```python
from build123d import *

# Parameters (mm, degrees)
SKETCH9_W           = 27.5
SKETCH9_H           = 28
BOSS_EXTRUDE2_DEPTH = 7.5
SKETCH10_W          = 23.5
SKETCH10_H          = 25.45
CUT_EXTRUDE1_DEPTH  = 6.1
SKETCH12_W          = 18.5
SKETCH12_H          = 12.3
CUT_EXTRUDE2_DEPTH  = 3
SKETCH11_W          = 9.585282086
SKETCH11_H          = 9.717675131
CUT_EXTRUDE3_DEPTH  = 5.05


with BuildPart() as part:
    # Sketch9 → Boss-Extrude2 (new, symmetric)
    with BuildSketch(Plane(origin=(0, 0, 0), x_dir=(1, 0, 0), z_dir=(0, 1, 0))):
        with Locations((0, 14)):
            Rectangle(SKETCH9_W, SKETCH9_H)
    extrude(amount=BOSS_EXTRUDE2_DEPTH, both=True)

    # Sketch10 → Cut-Extrude1 (cut, symmetric)
    with BuildSketch(Plane(origin=(0, 0, 0), x_dir=(1, 0, 0), z_dir=(0, 1, 0))):
        with Locations((0, 12.775)):
            Rectangle(SKETCH10_W, SKETCH10_H)
    extrude(amount=CUT_EXTRUDE1_DEPTH, both=True, mode=Mode.SUBTRACT)

    # Sketch12 → Cut-Extrude2 (cut)
    with BuildSketch(Plane.XY.offset(-28)):
        Rectangle(SKETCH12_W, SKETCH12_H)
    extrude(amount=CUT_EXTRUDE2_DEPTH, mode=Mode.SUBTRACT)

    # Sketch11 → Cut-Extrude3 (cut)
    with BuildSketch(Plane.XY.offset(5)):
        with Locations((8.957358957, -0.433824782)):
            Rectangle(SKETCH11_W, SKETCH11_H)
    extrude(amount=-CUT_EXTRUDE3_DEPTH, mode=Mode.SUBTRACT)


with BuildPart() as body_2:
    # Split1: the piece on the far side of the plane
    add(part.part)
    split(bisect_by=Plane.ZX, keep=Keep.BOTTOM)


with BuildPart() as part_1:
    add(part.part)

    # Split1
    split(bisect_by=Plane.ZX, keep=Keep.TOP)


solid = part_1.part
```
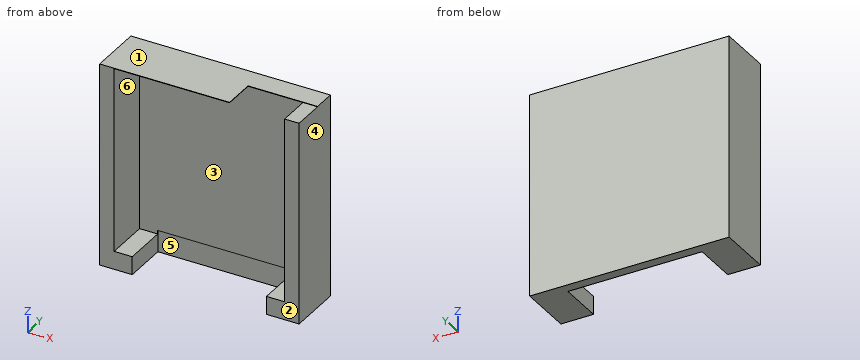
Check sheet for the modelled part. Datum: model origin and axes. Units: mm. Face numbers are marked on the shaded views. A direction names the side the tool comes from. Round coordinates to 2 decimals unless told otherwise and drop trailing zeros. Loops run counter-clockwise (first coordinate to the right, second up) from the corner with the lowest first, then second, coordinate; pieces in that order, holes last. Notation, with made-up numbers: (51, -29.75) -> (85, -29.75) arc R6 ccw to (85, -19.75) -> close; hole circle Ø6 at (1, -12). An arc over 180 degrees is marked (long way). Answer in a Markdown table with one row per item.
Q1. Release check for a two-part mould opening along Z. For the marked faces 1, 2 and 3 record: released by +Z, released by -Z, zero draft, split by the parting line, or undercut.
Data:
| item | result |
|---|---|
| face 1 | released by +Z |
| face 2 | zero draft |
| face 3 | undercut |
Q2. Thickness scan on L1, parallel to X at y = 4, z = -16.25; L2, parallel to Z at x = 10.75, y = 2; L3, parallel to Y at x = 1.75, z = -8.5. Record the ranges inside material, lowest first.
Data:
| item | result |
|---|---|
| L1 | x = -13.75 to -11.75, 11.75 to 13.75 |
| L2 | z = -28 to -25.5 |
| L3 | y = 6.1 to 7.5 |
Q3. Set-up check for the marked faces 4, 5 and 6: record each of +Z, -Z, +X, -X, +Y, -Y from which the full face is reachable in a straight line by a thin tool's end or side.
Data:
| item | result |
|---|---|
| face 4 | +Z, -Z, +X, +Y, -Y |
| face 5 | -Z, -Y |
| face 6 | -Y |
Q4. Sectioned sample at A-A on y = 4. Enter the section's corners in (x, z).
Data:
| item | result |
|---|---|
| outline | (-13.75, -28) -> (-9.25, -28) -> (-9.25, -25.5) -> (-11.75, -25.5) -> (-11.75, -0.05) -> (4.16, -0.05) -> (4.16, 0) -> (-13.75, 0) -> close; (9.25, -28) -> (13.75, -28) -> (13.75, -0.05) -> (11.75, -0.05) -> (11.75, -25.5) -> (9.25, -25.5) -> close |
Q5. Sectioned sample at C-C on z = -18.5. Enter the section's corners in (x, y).
Data:
| item | result |
|---|---|
| outline | (-13.75, 0) -> (-11.75, 0) -> (-11.75, 6.1) -> (11.75, 6.1) -> (11.75, 0) -> (13.75, 0) -> (13.75, 7.5) -> (-13.75, 7.5) -> close |
Q6. Go/stop test with flat-tipped pins: P1, Ø1.5, axis at x = 10.5, y = 2.5, coming from the +Z side; P2, Ø2, axis at x = -11, y = 3, coming from the +Z side; P3, Ø1.6, axis at x = 12.5, y = 1.5, coming from the +Z side; P4, Ø2, axis at x = 7, z = -7.5, coming from the -Y side. Record where each tip stops, or that it passes through.
Data:
| item | result |
|---|---|
| P1 | stops at z = -25.5 |
| P2 | stops at z = 0 |
| P3 | stops at z = -0.05 |
| P4 | stops at y = 6.1 |
Q7. Sectioned sample at B-B on x = -1.25. Enter the section's corners in (y, z), then the cut area to 3 significant figures.
Data:
| item | result |
|---|---|
| outline | (0, -0.05) -> (6.1, -0.05) -> (6.1, -25) -> (6.15, -25) -> (6.15, -28) -> (7.5, -28) -> (7.5, 0) -> (0, 0) -> close |
| area | 39.4 mm^2 |
